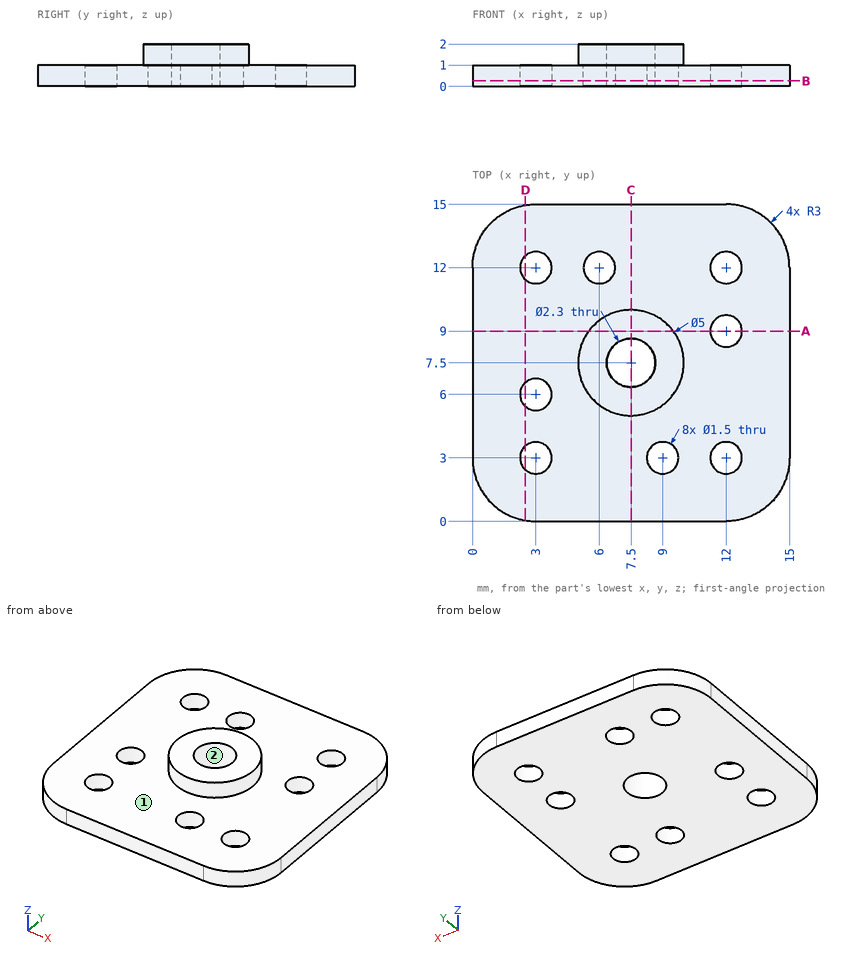
Job drawing, mm, ordinate dimensions from the low corner. One solid piece. Coordinates: 2 decimals unless noted, no trailing zeros. Order: outer loops, then holes, each group sorted by start corner. A loop starts at its lowest first (then second) coordinate and runs counter-clockwise, first axis right, second up. Notation, with made-up numbers: M 87,84.25 L 118,84.25 A22 ccw 118,105.25 Z; hole C -40,52.5 d10. An arc over 180 degrees is marked long. Answer as CSV lines item,"result".
(1) Pull direction Y, two halves, no side cores. Call the marked faces 1 and 2: +Y half, -Y half, draft (parallel to the pull), parting line (faces both ways), or undercut.
Geometry says:
face 1,"draft"
face 2,"undercut"
(2) Band-saw the part on C-C, the plane x = 7.5. List the corners of the cut face in (y, z), then the cut area to 3 significant figures.
Geometry says:
outline,"M 0,0 L 6.35,0 L 6.35,2 L 5,2 L 5,1 L 0,1 Z; M 8.65,0 L 15,0 L 15,1 L 10,1 L 10,2 L 8.65,2 Z"
area,"15.4 mm2"
(3) Wall check: line 1 along X through (y, z) = (3, 0.55); line 2 along Y through (x, z) = (6, 0.45); line 3 along Y through (x, z) = (7.5, 0.75). Give the ranges that are in metal, low to high.
Geometry says:
line 1,"x = 0 to 2.25, 3.75 to 8.25, 9.75 to 11.25, 12.75 to 15"
line 2,"y = 0 to 11.25, 12.75 to 15"
line 3,"y = 0 to 6.35, 8.65 to 15"
(4) Flat gauge pin, fed straight in: pin 1 (2.5 mm diameter, centred on x = 12, y = 3, fed in from +Z). Where does the tip first touch, or does it go through?
Geometry says:
pin 1,"stops at z = 1"
(5) Band-saw the part on B-B, the plane z = 0.25. State how many separate pieces and enclosed holes the cut face has, then the cut area to 3 significant figures.
Geometry says:
separate pieces,"1"
enclosed holes,"9"
area,"199 mm2"
(6) Band-saw the part on D-D, the plane x = 2.5. List the corners of the cut face in (y, z).
Geometry says:
outline,"M 0.04,0 L 2.44,0 L 2.44,1 L 0.04,1 Z; M 3.56,0 L 5.44,0 L 5.44,1 L 3.56,1 Z; M 6.56,0 L 11.44,0 L 11.44,1 L 6.56,1 Z; M 12.56,0 L 14.96,0 L 14.96,1 L 12.56,1 Z"
(7) Band-saw the part on A-A, the plane y = 9. List the corners of the cut face in (x, z), then the cut area to 3 significant figures.
Geometry says:
outline,"M 0,0 L 11.25,0 L 11.25,1 L 9.5,1 L 9.5,2 L 5.5,2 L 5.5,1 L 0,1 Z; M 12.75,0 L 15,0 L 15,1 L 12.75,1 Z"
area,"17.5 mm2"
